Geometry check sheet. Reference: the model listing, model coordinates, mm. Face numbers are marked on the shaded views. A direction names the side the tool comes from. Round coordinates to 2 decimals unless told otherwise and drop trailing zeros. Write each loop counter-clockwise with the first axis right and the second up, starting at its lowest first coordinate (ties: lowest second). Pieces come first, ordered by that corner, then holes. Notation, with made-up numbers: (79, 60) -> (89, 60) arc R20 cw to (89, 71) -> close; hole circle Ø11 at (2, 60.25). An arc over 180 degrees is marked (long way). Return JSON: item names as keys, results as strings. Group by question number.
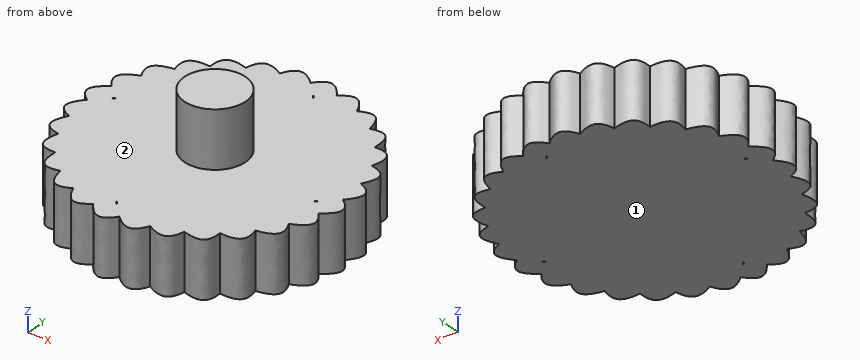
from build123d import *

# Parameters (mm, degrees)
F1_DEPTH = 25.4
F2_COUNT = 7
F3_R     = 5.08
F5_DEPTH = 25.4
F6_R     = 13.8422329742
F7_DEPTH = 25.4
F8_COUNT = 4


with BuildPart() as f1:
    # F0 (on Top) → F1 (new body)
    with BuildSketch(Plane.XY):
        with BuildLine():
            ThreePointArc((-0.3036099023, 41.7036828128), (-29.3821999901, -29.5968860332), (41.704787964, 0))
            ThreePointArc((41.704787964, 0), (38.5508515564, 15.909782632), (29.5660770028, 29.4132016242))
            ThreePointArc((29.5660770028, 29.4132016242), (15.869372299, 38.5675039633), (-0.3036099023, 41.7036828128))
        make_face()
        with BuildLine():
            ThreePointArc((-0.3036099023, 41.7036828128), (15.869372299, 38.5675039633), (29.5660770028, 29.4132016242))
            add(Edge.make_bspline(
                [(-0.3036099023, 41.7036828128), (6.4916545945, 50.8782567936), (20.9015792408, 70.3101588182), (26.5683495721, 43.5511495821), (29.5660770028, 29.4132016242)],
                knots=[0, 0, 0, 0, 0.4717280628, 1, 1, 1, 1], degree=3))
        make_face()
    extrude(amount=F1_DEPTH)

    # F2: F1 ×7 about axis
    f2_axis = Axis((0, 0, 25.4), (0, 0, -1))


with BuildPart() as f1_1:
    add(f1.part)
    for i in range(1, F2_COUNT):
        add(f1.part.rotate(f2_axis, i * 360 / F2_COUNT))

    # F3
    f3_edges = [f1_1.edges().sort_by_distance(p)[0] for p in [
        (-0.30361, 41.703683, 12.7),
    ]]
    fillet(f3_edges, radius=F3_R)

    # F4 (on face) → F5 (cut)
    with BuildSketch(Plane.XY.offset(25.4)):
        with BuildLine():
            add(Edge.make_bspline(
                [(-36.3872498274, -6.7111928947), (-41.8735206701, -9.5542377544), (-62.7340181989, 2.2079607061), (-29.4439624143, 18.5836450682), (-31.0447006553, -3.9426261585), (-36.3872498274, -6.7111928947)],
                knots=[0, 0, 0, 0, 0.3333906433, 0.6753430597, 1, 1, 1, 1], degree=3))
        make_face()
    extrude(amount=-F5_DEPTH, mode=Mode.SUBTRACT)

    # F6 (on face) → F7 (join)
    with BuildSketch(Plane.XY.offset(25.4)):
        Circle(F6_R)
    extrude(amount=F7_DEPTH)

    # F8: F1 ×4 about axis
    f8_axis = Axis((0, 0, 50.8), (0, 0, 1))


with BuildPart() as f1_2:
    add(f1_1.part)
    for i in range(1, F8_COUNT):
        add(f1_1.part.rotate(f8_axis, i * 360 / F8_COUNT))


solid = f1_2.part
1) Go/stop test with flat-tipped pins: P1, Ø1.5, axis at x = 26.5, y = 49, coming from the +Z side; P2, Ø5, axis at y = -7, z = 40.5, coming from the +X side; P3, Ø1, axis at y = 21.5, z = 15.5, coming from the -X side. Record where each tip stops, or that it passes through.
2) Tool access check on the marked faces 1 and 2. Record the directions out of +Z, -Z, +X, -X, +Y, -Y that give a thin tool (end or side, any length) a straight path to the whole face; none if there is none.
3) Material ranges on probe 1 along Y at (x, z) = (56.5, 24); probe 2 along Z at (x, y) = (-46.5, -11.5); probe 3 along Y at (x, z) = (13.5, 13.5), recorded low to high. Write a range as [from, to].
4) Sectioned sample at A-A on z = 45. Enter the section's corners in (x, y), and give its area (3 significant figures).
5) Sectioned sample at B-B on z = 10. State how many separate pieces and enclosed holes the cut face has, and give its area (3 significant figures).
Evaluation:
{
 "1": {"P1": "stops at z = 25.4", "P2": "stops at x = 13.09", "P3": "stops at x = -56.9"},
 "2": {"face 1": "-Z, +X, -X, +Y, -Y", "face 2": "+Z"},
 "3": {"probe 1": "y = [-21.31, -12.1], [-11.13, 13.46], [16.01, 23.74]", "probe 2": "z = [0, 25.4]", "probe 3": "y = [-56.41, 57.57]"},
 "4": {"outline": "circle Ø27.68 at (0, 0)", "area": "602 mm2"},
 "5": {"separate pieces": "1", "enclosed holes": "4", "area": "11,300 mm2"}
}
